The listing builds one solid part. Answer for the finished solid, in the listing's coordinates (mm). A direction names the side the tool comes from. Give positions to 0.01 mm unless a question says otherwise; leave off trailing zeros. Write each loop counter-clockwise with the first axis right and the second up, starting at its lowest first coordinate (ties: lowest second). Pieces come first, ordered by that corner, then holes. Notation, with made-up numbers: M 25.5,-3.5 L 57.5,-3.5 A24 ccw 57.5,9.5 Z; hole C 18,29 d7. An arc over 180 degrees is marked long. Answer as a JSON object with one key per item and string values.
```python
from build123d import *

# Parameters (mm, degrees)
F0_R     = 1.8
F0_W     = 26
F0_H     = 14
F1_DEPTH = 4
F0_H_2   = 4
F2_DEPTH = 29.6
F3_R     = 9.3
F4_DEPTH = 4
F5_R     = 3


with BuildPart() as f1:
    # F0 (on Top) → F1 (new body)
    with BuildSketch(Plane.XY):
        Polygon((0, 7.5), (-41, 7.5), (-41, 0), (-33.5, 0), (-7.5, 0), (0, 0), align=None)
        with Locations((-36, 3.75)):
            Circle(F0_R, mode=Mode.SUBTRACT)
        with Locations((-5, 3.75)):
            Circle(F0_R, mode=Mode.SUBTRACT)
        with Locations((-20.5, -7)):
            Rectangle(F0_W, F0_H)
    extrude(amount=F1_DEPTH)

    # F0 (on Top) → F2 (join)
    with BuildSketch(Plane.XY):
        with Locations((-20.5, -16)):
            Rectangle(F0_W, F0_H_2)
    extrude(amount=F2_DEPTH)

    # F3 (on face) → F4 (cut, through all)
    with BuildSketch(Plane(origin=(0, -14, 0), x_dir=(-1, 0, 0), z_dir=(0, 1, 0))):
        with Locations((20.5, 18.3)):
            Circle(F3_R)
    extrude(amount=-F4_DEPTH, mode=Mode.SUBTRACT)

    # F5
    f5_edges = [f1.edges().sort_by_distance(p)[0] for p in [
        (0, 0, 2),
        (0, 7.5, 2),
        (-41, 0, 2),
        (-41, 7.5, 2),
        (-33.5, -16, 29.6),
        (-7.5, -16, 29.6),
    ]]
    fillet(f5_edges, radius=F5_R)


solid = f1.part
```
1. Consider line 1 along Z through (x, y) = (-20.5, -16.05); line 2 along Y through (x, z) = (-36, 1.1); line 3 along Z through (x, y) = (-33, -1.25). Determine where each line is inside the solid, lowest interval first.
Verdict:
{"line 1": "z = 0 to 9, 27.6 to 29.6", "line 2": "y = 0 to 1.95, 5.55 to 7.5", "line 3": "z = 0 to 4"}
2. Flat-ended cylindrical pins translate along their axes: pin 1 (10 mm diameter, centred on x = -11, z = 21, fed in from +Y); pin 2 (3 mm diameter, centred on x = -5, y = 3.75, fed in from -Z); pin 3 (3 mm diameter, centred on y = -15, z = 11, fed in from +X); pin 4 (6.5 mm diameter, centred on x = -10.5, y = -5, fed in from +Z). Find the tip coordinate at first contact, or state that the pin passes through.
Verdict:
{"pin 1": "stops at y = -14", "pin 2": "passes through", "pin 3": "stops at x = -7.5", "pin 4": "stops at z = 4"}
3. A cutting plane is placed at C-C, the plane x = -5. Give the vertices of the cut face in (y, z), plus the area to 3 significant figures.
Verdict:
{"outline": "M 0,0 L 1.95,0 L 1.95,4 L 0,4 Z; M 5.55,0 L 7.5,0 L 7.5,4 L 5.55,4 Z", "area": "15.6 mm2"}
4. A cutting plane is placed at A-A, the plane z = 18.3. Give the vertices of the cut face in (x, y), plus the area to 3 significant figures.
Verdict:
{"outline": "M -33.5,-18 L -29.8,-18 L -29.8,-14 L -33.5,-14 Z; M -11.2,-18 L -7.5,-18 L -7.5,-14 L -11.2,-14 Z", "area": "29.6 mm2"}
5. The mould has two halves that part along X. Classify faces 4 (the cylindrical face through (-8.4, -15.97, 28.74)), 5 (the cylindrical face through (-40.1, 0.86, 2.03)), 6 (the cylindrical face through (-3.283, 4.291, 1.972)): released by +X, released by -X, zero draft, split by the parting line, or undercut.
Verdict:
{"face 4": "released by +X", "face 5": "released by -X", "face 6": "undercut"}
6. For faces 1 (the flat face through (-33.5, -14.4, 10.3)), 2 (the flat face through (-26.5, -14, 10.9)), 3 (the flat face through (-5, 0, 2)), determine the directions among +Z, -Z, +X, -X, +Y, -Y from which every point of the face is accessible in a straight line to the end or side of a thin tool.
Verdict:
{"face 1": "+Z, -Z, -X, -Y", "face 2": "+Z, +X, -X, +Y", "face 3": "+Z, -Z, +X, -Y"}
7. A cutting plane is placed at D-D, the plane y = 3.75. Give the vertices of the cut face in (x, z).
Verdict:
{"outline": "M -41,0 L -37.8,0 L -37.8,4 L -41,4 Z; M -34.2,0 L -6.8,0 L -6.8,4 L -34.2,4 Z; M -3.2,0 L 0,0 L 0,4 L -3.2,4 Z"}
8. A cutting plane is placed at B-B, the plane y = -16.25. Give the vertices of the cut face in (x, z), plus the area to 3 significant figures.
Verdict:
{"outline": "M -33.5,0 L -7.5,0 L -7.5,26.6 A3 ccw -10.5,29.6 L -30.5,29.6 A3 ccw -33.5,26.6 Z; hole C -20.5,18.3 d18.6", "area": "494 mm2"}
